from build123d import *

# Parameters (mm, degrees)
F0_W     = 38.1
F0_H     = 31.75
F1_DEPTH = 25.4
F3_DEPTH = 25.4


with BuildPart() as f1:
    # F0 (on Front) → F1 (new body)
    with BuildSketch(Plane.XZ):
        with Locations((19.05, 15.875)):
            Rectangle(F0_W, F0_H)
    extrude(amount=F1_DEPTH)

    # F2 (on face) → F3 (cut)
    with BuildSketch(Plane.YZ.offset(38.1)):
        Polygon((-25.4, 6.309687), (0, 31.75), (-8.660507, 31.75), (-25.4, 31.75), align=None)
    extrude(amount=-F3_DEPTH, mode=Mode.SUBTRACT)


solid = f1.part
Read the model definition and answer for the solid it produces. Units are mm, in the model's axes. A direction names the side the tool comes from. Coordinates: 2 decimals unless noted, no trailing zeros. Loops run counter-clockwise (first coordinate to the right, second up) from the corner with the lowest first, then second, coordinate; pieces in that order, holes last.
Q1. Which of the six approach directions +Z, -Z, +X, -X, +Y, -Y give full straight-line access (tool end or side, diameter ignored) to faces 1 (the face through (12.7, -16, 22)), 2 (the face through (19, -13, 0))?
Q2. The part is cut by section C-C on z = 22. Write down the section's boundary in (x, y).
Q3. The part is cut by section B-B on y = -5. Write down the section's boundary in (x, z), and give its area (3 significant figures).
Q4. Consider probe 1 along X at (y, z) = (-9.25, 28.5); probe 2 along Z at (x, y) = (20, -13.25); probe 3 along Y at (x, z) = (16, 27.5). Determine where each line is inside the solid, lowest interval first.
Q5. This flat-tipped pin is pushed along its axis until it touches: pin 1 Ø4 at (x, y) = (27.5, -20) entering from +Z. Where does it stop, or does it pass through?
Q6. The part is cut by section A-A on x = 33. Write down the section's boundary in (y, z).
Results below:
1. face 1: +Z, +X, -Y
1. face 2: -Z, +X, -X, +Y, -Y
2. outline: (0, -25.4) - (12.7, -25.4) - (12.7, -9.73) - (38.1, -9.73) - (38.1, 0) - (0, 0) - close
3. outline: (0, 0) - (38.1, 0) - (38.1, 26.74) - (12.7, 26.74) - (12.7, 31.75) - (0, 31.75) - close
3. area: 1,080 mm2
4. probe 1: x = 0 to 12.7
4. probe 2: z = 0 to 18.48
4. probe 3: y = -4.24 to 0
5. pin 1: stops at z = 13.72
6. outline: (-25.4, 0) - (0, 0) - (0, 31.75) - (-25.4, 6.31) - close
